Autodesk Inventor part; units mm, degrees
ref_plane "YZ Plane" through (0, 0, 0) normal (1, 0, 0) x (0, 1, 0)
ref_plane "XZ Plane" through (0, 0, 0) normal (0, 1, 0) x (-1, 0, 0)
ref_plane "XY Plane" through (0, 0, 0) normal (0, 0, 1) x (1, 0, 0)
sketch "Boceto1" plane through (0, 0, 0) normal (0, 0, 1) x (1, 0, 0)
  line L0 (5, -5) -> (165, -5)
  line L1 (165, -2.5) -> (8, -2.5)
  line L2 (8, -2.5) -> (8, 2.5)
  line L3 (8, 2.5) -> (165, 2.5)
  line L4 (140, 5) -> (142.5, 5)
  line L5 (142.5, 5) -> (137.5, 5)
  line L6 (137.5, 5) -> (137.5, 180)
  line L7 (142.5, 180) -> (142.5, 5)
  line L8 (132.5, 185) -> (147.5, 185)
  line L9 (147.5, 185) -> (147.5, 5)
  line L10 (142.5, 5) -> (137.5, 5)
  line L11 (132.5, 5) -> (132.5, 185)
  line L12 (137.5, 180) -> (142.5, 180)
  line L13 (147.5, 5) -> (165, 5)
  line L14 (0, 5) -> (132.5, 5)
  line L15 (137.5, 5) -> (142.5, 5)
  arc A0 (-165, 5) -> (-165, -5) centre (-165, 0) ccw
  line L16 (5, -5) -> (-165, -5)
  line L17 (-140, 5) -> (-142.5, 5)
  line L18 (-142.5, 5) -> (-137.5, 5)
  line L19 (-137.5, 5) -> (-137.5, 180)
  line L20 (-142.5, 180) -> (-142.5, 5)
  line L21 (-132.5, 185) -> (-147.5, 185)
  line L22 (-147.5, 185) -> (-147.5, 5)
  line L23 (-142.5, 5) -> (-137.5, 5)
  line L24 (-132.5, 5) -> (-132.5, 185)
  line L25 (-137.5, 180) -> (-142.5, 180)
  line L26 (-147.5, 5) -> (-165, 5)
  line L27 (0, 5) -> (-132.5, 5)
  line L28 (-137.5, 5) -> (-142.5, 5)
  line L29 (0, 0) -> (-5, 0) construction
  circle A1 centre (0, 0) radius 2.5
  arc A2 (180, -2.5) -> (180, 2.5) centre (180, 0) ccw
  line L30 (180, 5) -> (165, 5)
  line L31 (165, 2.5) -> (180, 2.5)
  line L32 (165, -2.5) -> (180, -2.5)
  line L33 (165, -5) -> (180, -5)
  arc A3 (180, -5) -> (180, 5) centre (180, 0) ccw
  dimension "d13" = 15
  dimension "d17" = 180
  dimension "d18" = 175
  dimension "d31" = 10
  dimension "d36" = 5
  dimension "d40" = 5
extrude "Extrusión1" add sketch "Boceto1" along normal blind 5
sketch "Sketch4" plane through (0, 0, 5) normal (0, 0, 1) x (1, 0, 0)
  line L0 (-132.5, 185) -> (-147.5, 185)
  line L1 (-132.5, 5) -> (-132.5, 185)
  line L2 (-147.5, 185) -> (-132.5, 185)
  line L3 (-132.5, 185) -> (-132.5, 180)
  line L4 (-132.5, 180) -> (-147.5, 180)
  line L5 (-147.5, 180) -> (-147.5, 185)
  line L6 (180, 5) -> (147.5, 5)
  line L7 (147.5, 5) -> (147.5, 185)
  line L8 (147.5, 185) -> (132.5, 185)
  line L9 (132.5, 185) -> (132.5, 5)
  line L10 (132.5, 5) -> (-132.5, 5)
  line L11 (-132.5, 5) -> (-132.5, 185)
  line L12 (-132.5, 185) -> (-147.5, 185)
  line L13 (-147.5, 185) -> (-147.5, 5)
  line L14 (-147.5, 5) -> (-165, 5)
  arc A0 (-165, 5) -> (-165, -5) centre (-165, 0) ccw
  line L15 (-165, -5) -> (180, -5)
  line L16 (-142.5, 5) -> (-142.5, 180)
  line L17 (-142.5, 180) -> (-137.5, 180)
  line L18 (-137.5, 180) -> (-137.5, 5)
  line L19 (-137.5, 5) -> (-142.5, 5)
  line L20 (142.5, 180) -> (142.5, 5)
  line L21 (142.5, 5) -> (137.5, 5)
  line L22 (137.5, 5) -> (137.5, 180)
  line L23 (137.5, 180) -> (142.5, 180)
  line L24 (132.5, 185) -> (147.5, 185)
  line L25 (147.5, 185) -> (147.5, 180)
  line L26 (147.5, 180) -> (132.5, 180)
  line L27 (132.5, 180) -> (132.5, 185)
  arc A1 (180, -5) -> (180, 5) centre (180, 0) ccw
  point P0 (0, 0)
  dimension "d26" = 5
extrude "Extrusion3" add sketch "Sketch4" along normal blind 10 contours L1 L4 L5 L0 | L9 L8 L7 L26 L23
sketch "Sketch5" plane through (0, 0, 5) normal (0, 0, 1) x (1, 0, 0)
  line L0 (180, -2.5) -> (8, -2.5)
  line L1 (8, -2.5) -> (8, 2.5)
  line L2 (8, 2.5) -> (180, 2.5)
  arc A0 (180, -2.5) -> (180, 2.5) centre (180, 0) ccw
  circle A1 centre (0, 0) radius 2.5
  line L3 (147.5, 180) -> (142.5, 180)
  line L4 (142.5, 180) -> (142.5, 5)
  line L5 (142.5, 5) -> (137.5, 5)
  line L6 (137.5, 5) -> (137.5, 180)
  line L7 (137.5, 180) -> (132.5, 180)
  line L8 (132.5, 180) -> (132.5, 5)
  line L9 (132.5, 5) -> (-132.5, 5)
  line L10 (-132.5, 5) -> (-132.5, 180)
  line L11 (-132.5, 180) -> (-137.5, 180)
  line L12 (-137.5, 180) -> (-137.5, 5)
  line L13 (-137.5, 5) -> (-142.5, 5)
  line L14 (-142.5, 5) -> (-142.5, 180)
  line L15 (-142.5, 180) -> (-147.5, 180)
  line L16 (-147.5, 180) -> (-147.5, 5)
  line L17 (-147.5, 5) -> (-165, 5)
  arc A2 (-165, 5) -> (-165, -5) centre (-165, 0) ccw
  line L18 (-165, -5) -> (180, -5)
  arc A3 (180, -5) -> (180, 5) centre (180, 0) ccw
  line L19 (180, 5) -> (147.5, 5)
  line L20 (147.5, 5) -> (147.5, 180)
  arc A4 (-165, 5) -> (-165, -5) centre (-165, 0) ccw
  line L21 (-165, -5) -> (-185, -5)
  line L22 (-185, -5) -> (-185, 5)
  line L23 (-185, 5) -> (-165, 5)
  line L24 (-165, 5) -> (-165, -5)
  arc A5 (180, -5) -> (180, 5) centre (180, 0) ccw
  line L25 (180, 5) -> (200, 5)
  line L26 (200, 5) -> (200, -5)
  line L27 (200, -5) -> (180, -5)
  dimension "d42" = 20
  dimension "d45" = 20
extrude "Extrusion4" add sketch "Sketch5" against normal up to surface (5 mm away) contours L25 L26 L27 A3 | L21 L22 L23 A2 | A2 L24
sketch "Sketch6" plane through (0, 0, 5) normal (0, 0, 1) x (1, 0, 0)
  line L0 (-147.5, 180) -> (-132.5, 180)
  line L1 (-132.5, 180) -> (-132.5, 185)
  line L2 (-132.5, 185) -> (-147.5, 185)
  line L3 (-147.5, 185) -> (-147.5, 180)
  line L4 (-147.5, 5) -> (-185, 5)
  line L5 (200, -5) -> (-185, -5)
  line L6 (-185, 5) -> (-180, 5)
  line L7 (-180, 5) -> (-180, -5)
  line L8 (-180, -5) -> (-185, -5)
  line L9 (-185, -5) -> (-185, 5)
  line L10 (200, -5) -> (200, 5)
  line L11 (200, 5) -> (195, 5)
  line L12 (195, 5) -> (195, -5)
  line L13 (195, -5) -> (200, -5)
  line L14 (200, -5) -> (200, 5)
  point P0 (0, 0)
  dimension "d46" = 15
  dimension "d47" = 5
  dimension "d48" = 5
  dimension "d49" = 5
  dimension "d50" = 10
extrude "Extrusion5" add sketch "Sketch6" along normal up to surface (10 mm away) contours L7 L5 L9 L4 | L12 L11 L10 L5
sketch "Sketch7" plane through (-185, -5, 0) normal (-1, 0, 0) x (0, 0, 1)
  line L0 (15, 0) -> (15, 10)
  line L1 (0, 0) -> (15, 0)
  line L2 (15, 10) -> (10, 10)
  line L3 (10, 10) -> (10, 0)
  line L4 (10, 0) -> (15, 0)
  line L5 (15, 0) -> (15, 10)
  point P0 (0, 5)
  dimension "d53" = 5
extrude "Extrusion6" add sketch "Sketch7" along normal blind 10
sketch "Sketch8" plane through (200, -5, 0) normal (1, 0, 0) x (0, 0, -1)
  line L0 (-10, 10) -> (-10, 0)
  line L1 (-10, 0) -> (-15, 0)
  line L2 (-15, 0) -> (-15, 10)
  line L3 (-15, 10) -> (-10, 10)
  point P0 (0, 5)
extrude "Extrusion7" add sketch "Sketch8" along normal blind 10
sketch "Sketch9" plane through (-180, -5, 15) normal (0, 0, 1) x (1, 0, 0)
  line L0 (32.5, 10) -> (-5, 10)
  line L1 (0, 0) -> (375, 0)
  line L2 (-5, 0) -> (-5, 10)
  line L3 (0, 0) -> (-15, 0)
  line L4 (0, 10) -> (0, 0)
  line L5 (0, 10) -> (-15, 10)
  line L6 (-15, 0) -> (-15, 10)
  line L7 (-15, 10) -> (-5, 10) construction
  line L8 (-5, 10) -> (-5, 0) construction
  line L9 (-5, 0) -> (-15, 0) construction
  line L10 (-15, 0) -> (-15, 10) construction
  circle A0 centre (-10, 5) radius 1.5
  line L11 (375, 10) -> (390, 10)
  line L12 (375, 0) -> (375, 10)
  line L13 (375, 0) -> (390, 0)
  line L14 (390, 10) -> (390, 0)
  line L15 (380, 10) -> (380, 0)
  line L16 (327.5, 10) -> (380, 10) construction
  line L17 (375, 0) -> (390, 0) construction
  line L18 (380, 10) -> (390, 10) construction
  line L19 (390, 10) -> (390, 0) construction
  line L20 (390, 0) -> (380, 0) construction
  line L21 (380, 0) -> (380, 10) construction
  circle A1 centre (385, 5) radius 1.5
  point P0 (180, 5)
  dimension "d58" = 3
  dimension "d61" = 3
extrude "Extrusion8" cut sketch "Sketch9" against normal blind 10 contours A0 | A1
sketch "Sketch10" plane through (-147.5, 185, 0) normal (0, 1, 0) x (1, 0, 0)
  line L0 (342.5, -5) -> (295, -5)
  line L1 (295, -5) -> (290, -5)
  line L2 (290, -5) -> (285, -5)
  line L3 (285, -5) -> (280, -5)
  line L4 (280, -5) -> (15, -5)
  line L5 (15, -5) -> (10, -5)
  line L6 (10, -5) -> (5, -5)
  line L7 (5, -5) -> (0, -5)
  line L8 (0, -5) -> (-32.5, -5)
  line L9 (-32.5, -5) -> (342.5, -5)
  line L10 (150, -5) -> (145, -5)
  line L11 (327.5, -5) -> (155.5, -5)
  line L12 (155.5, -5) -> (327.5, -5)
  line L13 (327.5, -5) -> (327.5, -5)
  line L14 (15, 0) -> (15, -15) construction
  line L15 (0, -5) -> (15, -5) construction
  line L16 (15, -5) -> (15, -15) construction
  line L17 (15, -15) -> (0, -15) construction
  line L18 (0, -15) -> (0, -5) construction
  line L19 (295, 0) -> (295, -15) construction
  line L20 (295, -15) -> (280, -15) construction
  line L21 (280, -15) -> (280, -5) construction
  line L22 (280, -5) -> (295, -5) construction
  line L23 (295, -5) -> (295, -15) construction
  circle A0 centre (7.5, -10) radius 1.5
  circle A1 centre (287.5, -10) radius 1.5
  point P0 (147.5, 0)
  dimension "d62" = 3
  dimension "d63" = 3
extrude "Extrusion9" cut sketch "Sketch10" against normal blind 10
properties part number "Bancada"
Work out the finished part from the listing and answer in its coordinate system (mm). A direction names the side the tool comes from. Round coordinates to 2 decimals unless told otherwise and drop trailing zeros. Write each loop counter-clockwise with the first axis right and the second up, starting at its lowest first coordinate (ties: lowest second). Pieces come first, ordered by that corner, then holes. Notation, with made-up numbers: (-24.75, 15) - (19.25, 15) arc R21 ccw to (19.25, 32) - close; hole circle Ø10 at (83, -27). An arc over 180 degrees is marked (long way). Return JSON: item names as keys, results as strings. Group by question number.
Q1. Find the intervals of material crossed by L1, parallel to X at y = 147, z = 4.5; L2, parallel to X at y = 183.6, z = 10; L3, parallel to Y at x = -190, z = 13.9, in increasing order.
Q2. The part is cut by section B-B on z = 2.5. Write down the section's boundary in (x, y), then the cut area to 3 significant figures.
Q3. The part is cut by section A-A on y = 81. Write down the section's boundary in (x, z).
Q4. The part is cut by section C-C on x = -59.5. Write down the section's boundary in (y, z), then the cut area to 3 significant figures.
Q5. The mould has two halves that part along Y. Classify faces 6 (the flat face through (7, -5, 4)), 7 (the flat face through (140, 180, 7)), 8 (the flat face through (-185, 0, 5)): released by +Y, released by -Y, zero draft, split by the parting line, or undercut.
Q6. For faces 1 (the flat face through (-140, 180, 7)), 2 (the flat face through (200, 0, 5)), 3 (the flat face through (-147.5, 102, 4)), 4 (the flat face through (185, 5, 4)), 5 (the flat face through (-132.5, 101, 4)), determine the directions among +Z, -Z, +X, -X, +Y, -Y from which every point of the face is accessible in a straight line to the end or side of a thin tool.
Q7. Each of these flat-tipped pins is pushed along its axis until it touches: pin 1 Ø8 at (y, z) = (0, 8) entering from -X; pin 2 Ø4 at (y, z) = (59, 2.5) entering from +X; pin 3 Ø3 at (x, y) = (-190.5, -0.5) entering from -Z; pin 4 Ø5.5 at (x, z) = (96, 2.5) entering from +Y. Where does it stop, or does it pass through?
Solved:
{
 "1": {"L1": "-147.5 to -142.5, -137.5 to -132.5, 132.5 to 137.5, 142.5 to 147.5", "L2": "-147.5 to -141.5, -138.5 to -132.5, 132.5 to 138.5, 141.5 to 147.5", "L3": "-5 to -1.5, 1.5 to 5"},
 "2": {"outline": "(-185, -5) - (200, -5) - (200, 5) - (147.5, 5) - (147.5, 185) - (132.5, 185) - (132.5, 5) - (-132.5, 5) - (-132.5, 185) - (-147.5, 185) - (-147.5, 5) - (-185, 5) - close; hole (-142.5, 5) - (-137.5, 5) - (-137.5, 180) - (-142.5, 180) - close; hole circle Ø5 at (0, 0); hole (8, -2.5) - (180, -2.5) arc R2.5 ccw to (180, 2.5) - (8, 2.5) - close; hole (137.5, 5) - (142.5, 5) - (142.5, 180) - (137.5, 180) - close", "area": "6,610 mm²"},
 "3": {"outline": "(-147.5, 0) - (-142.5, 0) - (-142.5, 5) - (-147.5, 5) - close; (-137.5, 0) - (-132.5, 0) - (-132.5, 5) - (-137.5, 5) - close; (132.5, 0) - (137.5, 0) - (137.5, 5) - (132.5, 5) - close; (142.5, 0) - (147.5, 0) - (147.5, 5) - (142.5, 5) - close"},
 "4": {"outline": "(-5, 0) - (5, 0) - (5, 5) - (-5, 5) - close", "area": "50.0 mm²"},
 "5": {"face 6": "released by -Y", "face 7": "undercut", "face 8": "zero draft"},
 "6": {"face 1": "+Z", "face 2": "-Z, +X, +Y, -Y", "face 3": "+Z, -Z, -X, +Y", "face 4": "+Z, -Z, +X, +Y", "face 5": "+Z, -Z, +Y"},
 "7": {"pin 1": "x = -195", "pin 2": "x = 147.5", "pin 3": "z = 10", "pin 4": "y = 5"}
}
